from build123d import *

# Parameters (mm, degrees)
F0_R     = 88.9
F0_W     = 127
F0_H     = 508
F1_DEPTH = 25.4
F2_W     = 25.4
F2_H     = 12.7
F2_H_2   = 292.1
F2_H_3   = 304.8
F2_H_4   = 203.2
F3_DEPTH = 127


with BuildPart() as f1:
    # F0 (on Top) → F1 (new body)
    with BuildSketch(Plane.XY):
        with BuildLine():
            ThreePointArc((-1000.085346, 739.070513), (-947.597523, 701.69854), (-892.846368, 667.728745))
            ThreePointArc((-892.846368, 667.728745), (-784.551405, 650.728892), (-692.86208, 710.811016))
            Line((-692.86208, 710.811016), (-88.9, 710.811016))
            Line((-88.9, 710.811016), (-88.9, 508))
            Line((-88.9, 508), (-342.9, 254))
            Line((-342.9, 254), (-342.9, -508))
            Line((-342.9, -508), (-88.9, -508))
            Line((-88.9, -508), (-88.9, -710.811016))
            Line((-88.9, -710.811016), (-692.86208, -710.811016))
            ThreePointArc((-692.86208, -710.811016), (-784.551405, -650.728892), (-892.846368, -667.728745))
            ThreePointArc((-892.846368, -667.728745), (-947.597523, -701.69854), (-1000.085346, -739.070513))
            ThreePointArc((-1000.085346, -739.070513), (-1030.142423, -799.711016), (-1000.085346, -860.35152))
            ThreePointArc((-1000.085346, -860.35152), (-947.597523, -897.723493), (-892.846368, -931.693288))
            ThreePointArc((-892.846368, -931.693288), (-784.551405, -948.693141), (-692.86208, -888.611016))
            Line((-692.86208, -888.611016), (692.86208, -888.611016))
            ThreePointArc((692.86208, -888.611016), (784.551405, -948.693141), (892.846368, -931.693288))
            ThreePointArc((892.846368, -931.693288), (947.597523, -897.723493), (1000.085346, -860.35152))
            ThreePointArc((1000.085346, -860.35152), (1030.142423, -799.711016), (1000.085346, -739.070513))
            ThreePointArc((1000.085346, -739.070513), (947.597523, -701.69854), (892.846368, -667.728745))
            ThreePointArc((892.846368, -667.728745), (784.551405, -650.728892), (692.86208, -710.811016))
            Line((692.86208, -710.811016), (88.9, -710.811016))
            Line((88.9, -710.811016), (88.9, -508))
            Line((88.9, -508), (342.9, -508))
            Line((342.9, -508), (342.9, 254))
            Line((342.9, 254), (88.9, 508))
            Line((88.9, 508), (88.9, 710.811016))
            Line((88.9, 710.811016), (692.86208, 710.811016))
            ThreePointArc((692.86208, 710.811016), (784.551405, 650.728892), (892.846368, 667.728745))
            ThreePointArc((892.846368, 667.728745), (947.597523, 701.69854), (1000.085346, 739.070513))
            ThreePointArc((1000.085346, 739.070513), (1030.142423, 799.711016), (1000.085346, 860.35152))
            ThreePointArc((1000.085346, 860.35152), (947.597523, 897.723493), (892.846368, 931.693288))
            ThreePointArc((892.846368, 931.693288), (784.551405, 948.693141), (692.86208, 888.611016))
            Line((692.86208, 888.611016), (-692.86208, 888.611016))
            ThreePointArc((-692.86208, 888.611016), (-784.551405, 948.693141), (-892.846368, 931.693288))
            ThreePointArc((-892.846368, 931.693288), (-947.597523, 897.723493), (-1000.085346, 860.35152))
            ThreePointArc((-1000.085346, 860.35152), (-1030.142423, 799.711016), (-1000.085346, 739.070513))
        make_face()
        with Locations((-816.646368, -799.711016)):
            Circle(F0_R, mode=Mode.SUBTRACT)
        with Locations((-127, 0)):
            Rectangle(F0_W, F0_H, mode=Mode.SUBTRACT)
        with Locations((816.646368, -799.711016)):
            Circle(F0_R, mode=Mode.SUBTRACT)
        with Locations((127, 0)):
            Rectangle(F0_W, F0_H, mode=Mode.SUBTRACT)
        with Locations((-816.646368, 799.711016)):
            Circle(F0_R, mode=Mode.SUBTRACT)
        with Locations((816.646368, 799.711016)):
            Circle(F0_R, mode=Mode.SUBTRACT)
    extrude(amount=F1_DEPTH)

    # F2 (on face) → F3 (join)
    with BuildSketch(Plane.XY.offset(25.4)):
        with Locations((-279.4, -6.35)):
            Rectangle(F2_W, F2_H)
        with Locations((-279.4, 146.05)):
            Rectangle(F2_W, F2_H_2)
        with Locations((279.4, 139.7)):
            Rectangle(F2_W, F2_H_3)
        with Locations((279.4, -165.1)):
            Rectangle(F2_W, F2_H_4)
    extrude(amount=F3_DEPTH)


solid = f1.part
Check sheet for the modelled part. Datum: model origin and axes. Units: mm. A direction names the side the tool comes from. Round coordinates to 2 decimals unless told otherwise and drop trailing zeros. Write each loop counter-clockwise with the first axis right and the second up, starting at its lowest first coordinate (ties: lowest second). Pieces come first, ordered by that corner, then holes. Notation, with made-up numbers: (85, 73) - (104, 73) arc R12 ccw to (104, 93) - close; hole circle Ø6 at (74, -22.75). An arc over 180 degrees is marked (long way). Return JSON: item names as keys, results as strings.
Q1. Cross-section at C-C (y = -196). Record the boundary of the cut face in (x, z), then the cut area to 3 significant figures.
Returned:
{"outline": "(-342.9, 0) - (-190.5, 0) - (-190.5, 25.4) - (-342.9, 25.4) - close; (-63.5, 0) - (63.5, 0) - (63.5, 25.4) - (-63.5, 25.4) - close; (190.5, 0) - (342.9, 0) - (342.9, 25.4) - (292.1, 25.4) - (292.1, 152.4) - (266.7, 152.4) - (266.7, 25.4) - (190.5, 25.4) - close", "area": "14,200 mm²"}
Q2. Draft check along X on faces 6 (the cylindrical face through (-783.018, 948.355, 12.522)), 7 (the flat face through (266.7, -167, 88)), 8 (the cylindrical face through (948.35, -702.2, 12.52)). Enter one of: released by +X, released by -X, zero draft, split by the parting line, or undercut.
Returned:
{"face 6": "undercut", "face 7": "released by -X", "face 8": "released by +X"}
Q3. Scan lines: L1, parallel to X at y = -707, z = 22; L2, parallel to X at y = 11, z = 21; L3, parallel to Z at x = -23, y = 516. Record each from-to range of solid material in increasing order. Write a range as from..to.
Returned:
{"L1": "x = -955.49..-695.69, -88.9..88.9, 695.69..955.49", "L2": "x = -342.9..-190.5, -63.5..63.5, 190.5..342.9", "L3": "z = 0..25.4"}
Q4. Depth check by flat-ended pin: P1, Ø20.5, axis at x = -273.5, z = 58.5, coming from the +Y side; P2, Ø3, axis at y = -85, z = 134.5, coming from the +X side; P3, Ø7.5, axis at x = 262.5, z = 7, coming from the +Y side. Enter the tip coordinate at first touch or a pass-through.
Returned:
{"P1": "stops at y = 292.1", "P2": "stops at x = 292.1", "P3": "stops at y = 888.61"}
Q5. Cross-section at A-A (x = 153). Record the boundary of the cut face in (y, z).
Returned:
{"outline": "(-888.61, 0) - (-710.81, 0) - (-710.81, 25.4) - (-888.61, 25.4) - close; (-508, 0) - (-254, 0) - (-254, 25.4) - (-508, 25.4) - close; (254, 0) - (443.9, 0) - (443.9, 25.4) - (254, 25.4) - close; (710.81, 0) - (888.61, 0) - (888.61, 25.4) - (710.81, 25.4) - close"}
Q6. Access from +Z, -Z, +X, -X, +Y, -Y to the whole of each face (thin tool, end or side, straight path). Record for faces 1 (the cylindrical face through (-946.85, -701.2, 12.52)), 2 (the cylindrical face through (783.018, 651.067, 12.522)), 3 (the flat face through (266.7, 138, 88)), 4 (the flat face through (217.7, 379.2, 12.5)), 5 (the flat face through (292.1, 138, 88)).
Returned:
{"face 1": "+Z, -Z, -X", "face 2": "+Z, -Z", "face 3": "+Z, +Y, -Y", "face 4": "+Z, -Z, +X", "face 5": "+Z, +X, +Y, -Y"}
Q7. Cross-section at B-B (z = 51.5). Record the boundary of the cut face in (x, y), then the cut area to 3 significant figures.
Returned:
{"outline": "(-292.1, -12.7) - (-266.7, -12.7) - (-266.7, 292.1) - (-292.1, 292.1) - close; (266.7, -266.7) - (292.1, -266.7) - (292.1, -63.5) - (266.7, -63.5) - close; (266.7, -12.7) - (292.1, -12.7) - (292.1, 292.1) - (266.7, 292.1) - close", "area": "20,600 mm²"}
Q8. Cross-section at D-D (x = 592). Record the boundary of the cut face in (y, z).
Returned:
{"outline": "(-888.61, 0) - (-710.81, 0) - (-710.81, 25.4) - (-888.61, 25.4) - close; (710.81, 0) - (888.61, 0) - (888.61, 25.4) - (710.81, 25.4) - close"}
